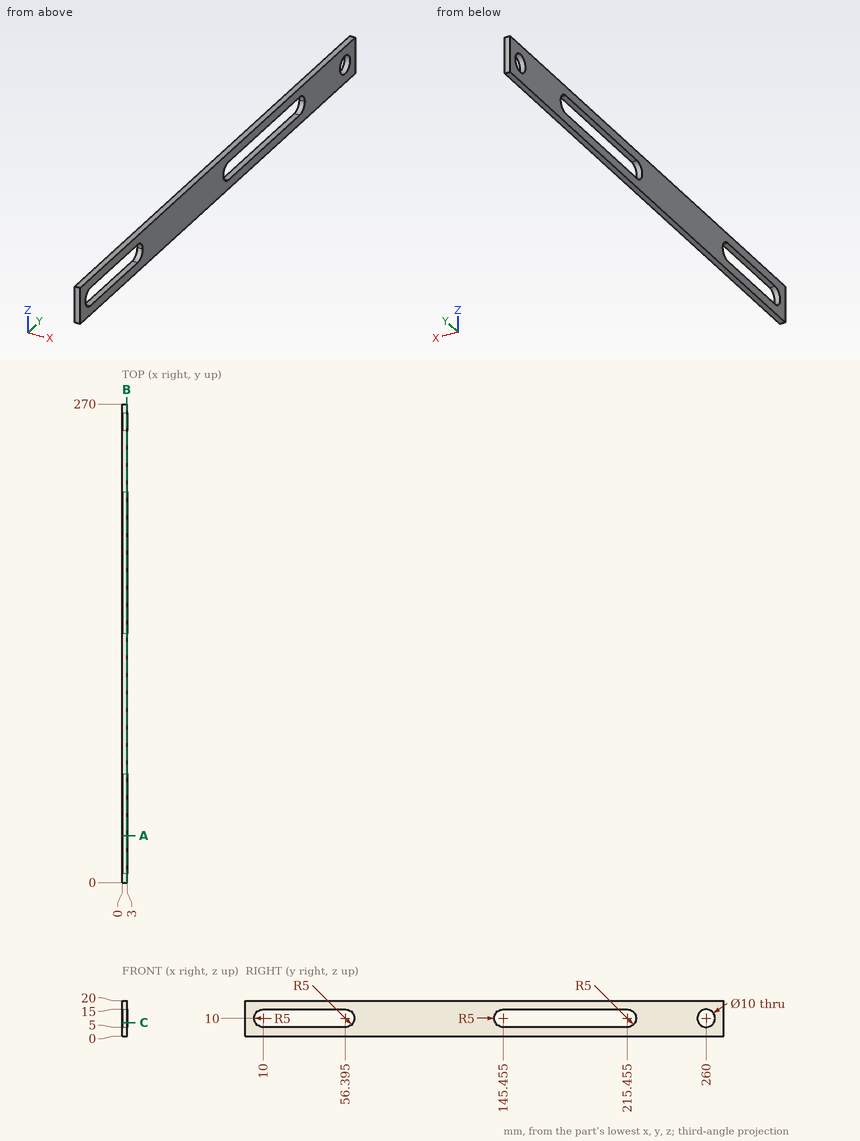
Design review of the part shown in the three views and the two pictorial views. Dimensions are in mm from the part's minimum x, y and z. Coordinates: 2 decimals unless noted, no trailing zeros. Loops run counter-clockwise (first coordinate to the right, second up) from the corner with the lowest first, then second, coordinate; pieces in that order, holes last.
(1) Consider section A-A, the plane y = 26.5. Give the boundary of the cut face in (x, z).
Determined:
outline: (0, 0) - (3, 0) - (3, 5) - (0, 5) - close; (0, 15) - (3, 15) - (3, 20) - (0, 20) - close
(2) Consider section B-B, the plane x = 2.55. Give the boundary of the cut face in (y, z) (1 decimal).
Determined:
outline: (0, 0) - (270, 0) - (270, 20) - (0, 20) - close; hole (10, 5) - (56.4, 5) arc R5 ccw to (56.4, 15) - (10, 15) arc R5 ccw to start; hole (145.5, 5) - (215.5, 5) arc R5 ccw to (215.5, 15) - (145.5, 15) arc R5 ccw to start; hole circle Ø10 at (260, 10)
(3) Wall thickness on L1, parallel to Y at x = 2.5, z = 9.75; L2, parallel to Z at x = 0.8, y = 260; L3, parallel to Y at x = 0.25, z = 6.5 (1 decimal): over which ranges is each line inside the solid? List them lowest first.
Determined:
L1: y = 0 to 5.01, 61.39 to 140.46, 220.45 to 255.01, 264.99 to 270
L2: z = 0 to 5, 15 to 20
L3: y = 0 to 6.4, 60 to 141.9, 219 to 256.4, 263.6 to 270
(4) Consider section C-C, the plane z = 7.5. Give the boundary of the cut face in (x, y) (1 decimal), plus the area to 3 significant figures.
Determined:
outline: (0, 0) - (3, 0) - (3, 5.7) - (0, 5.7) - close; (0, 60.7) - (3, 60.7) - (3, 141.1) - (0, 141.1) - close; (0, 219.8) - (3, 219.8) - (3, 255.7) - (0, 255.7) - close; (0, 264.3) - (3, 264.3) - (3, 270) - (0, 270) - close
area: 383 mm2
